from build123d import *

# Parameters (mm, degrees)
F0_R     = 4.7625
F1_DEPTH = 3.175


with BuildPart() as f1:
    # F0 (on Front) → F1 (new body)
    with BuildSketch(Plane.XZ):
        with BuildLine():
            ThreePointArc((42.829464, 11.355551), (22.018453, 22.018453), (11.355551, 42.829464))
            ThreePointArc((11.355551, 42.829464), (5.253764, 47.606357), (0, 41.91))
            Line((0, 41.91), (0, 12.7))
            ThreePointArc((0, 12.7), (3.719744, 3.719744), (12.7, 0))
            Line((12.7, 0), (41.91, 0))
            ThreePointArc((41.91, 0), (47.606357, 5.253764), (42.829464, 11.355551))
        make_face()
        with Locations((12.7, 12.7)):
            Circle(F0_R, mode=Mode.SUBTRACT)
        with Locations((28.575, 7.62)):
            Circle(F0_R, mode=Mode.SUBTRACT)
        with Locations((7.62, 29.845)):
            Circle(F0_R, mode=Mode.SUBTRACT)
    extrude(amount=F1_DEPTH)


solid = f1.part
The listing builds one solid part. Answer for the finished solid, in the listing's coordinates (mm). Round coordinates to 2 decimals unless told otherwise and drop trailing zeros. Order: outer loops, then holes, each group sorted by start corner. A loop starts at its lowest first (then second) coordinate and runs counter-clockwise, first axis right, second up. Notation, with made-up numbers: M 21.25,75.5 L 78.25,75.5 A18 cw 78.25,93.5 Z; hole C 2.25,26.5 d9. An arc over 180 degrees is marked long. Answer in a Markdown table with one row per item. Add a question column.
1) The part is cut by section B-B on z = 29. Determine the outline of the cut face in (x, y) (3 decimals), plus the area to 3 significant figures.
2) The part is cut by section A-A on x = 14. Determine the outline of the cut face in (y, z) (3 decimals), plus the area to 3 significant figures.
3) The part is cut by section C-C on y = -2.6. Determine the outline of the cut face in (x, z) (1 decimal), plus the area to 3 significant figures.
4) The part is cut by section D-D on z = 21.5. Determine the outline of the cut face in (x, y) (3 decimals).
5) Flat-ended cylindrical pins translate along their axes: pin 1 Ø1.5 at (x, y) = (7.5, -2.5) entering from +Z; pin 2 Ø8.5 at (x, z) = (12.7, 12.7) entering from +Y. Find the tip coordinate at first contact, or state that the pin passes through.
6) Consider line 1 along X through (y, z) = (-2.5, 8.5); line 2 along Z through (x, y) = (9, -2.55); line 3 along Z through (x, y) = (14, -2.9). Determine where each line is inside the solid, lowest interval first. Write a range as from..to.
7) Determine the mould class of faces 1 (the face through (7.942, -1.565, 12.909)), 2 (the face through (5.373, -1.565, 47.615)), 3 (the face through (27, -2, 0)) for opening direction X: pulls with the +X half, pulls with the -X half, needs draft (parallel to the pull), parting line crosses it, or undercut.
Findings below:
| question | item | result |
|---|---|---|
| 1 | outline | M 0,-3.175 L 2.933,-3.175 L 2.933,0 L 0,0 Z; M 12.307,-3.175 L 16.506,-3.175 L 16.506,0 L 12.307,0 Z |
| 1 | area | 22.6 mm² |
| 2 | outline | M -3.175,0 L 0,0 L 0,8.118 L -3.175,8.118 Z; M -3.175,17.282 L 0,17.282 L 0,33.811 L -3.175,33.811 Z |
| 2 | area | 78.3 mm² |
| 3 | outline | M 0,12.7 A12.7 ccw 12.7,0 L 41.9,0 A5.7 ccw 42.8,11.4 A38.1 cw 11.4,42.8 A5.7 ccw 0,41.9 Z; hole C 7.6,29.8 d9.5; hole C 12.7,12.7 d9.5; hole C 28.6,7.6 d9.5 |
| 3 | area | 955 mm² |
| 4 | outline | M 0,-3.175 L 22.547,-3.175 L 22.547,0 L 0,0 Z |
| 5 | pin 1 | stops at z = 47.53 |
| 5 | pin 2 | passes through |
| 6 | line 1 | x = 0.71..10.45, 14.95..23.89, 33.26..46.9 |
| 6 | line 2 | z = 0.55..9.7, 15.7..25.29, 34.4..46.59 |
| 6 | line 3 | z = 0..8.12, 17.28..33.81 |
| 7 | face 1 | undercut |
| 7 | face 2 | parting line crosses it |
| 7 | face 3 | needs draft |
